Read the model definition and answer for the solid it produces. Units are mm, in the model's axes. A direction names the side the tool comes from. Coordinates: 2 decimals unless noted, no trailing zeros. Write each loop counter-clockwise with the first axis right and the second up, starting at its lowest first coordinate (ties: lowest second). Pieces come first, ordered by that corner, then holes. Notation, with made-up numbers: (-16, 69) - (30, 69) arc R28 ccw to (30, 96) - close; hole circle Ø8 at (86, -33.75). An arc over 180 degrees is marked (long way). Return JSON: item names as keys, results as strings.
```python
from build123d import *

# Parameters (mm, degrees)
SKETCH1_R           = 17.25
BOSS_EXTRUDE1_DEPTH = 4.5
SKETCH2_R           = 2
CUT_EXTRUDE1_DEPTH  = 9
SKETCH3_R           = 14.7
SKETCH3_R_2         = 6
CUT_EXTRUDE2_DEPTH  = 7
CUT_EXTRUDE3_REACH  = 4
SKETCH4_R           = 3
SKETCH5_R           = 1.35933313
CUT_EXTRUDE4_DEPTH  = 18


with BuildPart() as part:
    # Sketch1 → Boss-Extrude1 (new body, symmetric)
    with BuildSketch(Plane.XY):
        Circle(SKETCH1_R)
    extrude(amount=BOSS_EXTRUDE1_DEPTH, both=True)

    # Sketch2 → Cut-Extrude1 (cut)
    with BuildSketch(Plane.XY.offset(4.5)):
        Circle(SKETCH2_R)
    extrude(amount=-CUT_EXTRUDE1_DEPTH, mode=Mode.SUBTRACT)

    # Sketch3 → Cut-Extrude2 (cut)
    with BuildSketch(Plane.XY.offset(4.5)):
        Circle(SKETCH3_R)
        Circle(SKETCH3_R_2, mode=Mode.SUBTRACT)
    extrude(amount=-CUT_EXTRUDE2_DEPTH, mode=Mode.SUBTRACT)

    # Sketch4 → Cut-Extrude3 (cut, up to next)
    with BuildSketch(Plane.XY.offset(-2.5), mode=Mode.PRIVATE) as cut_extrude3_sk1:
        with Locations((10.5, 0)):
            Circle(SKETCH4_R)
    cut_extrude3_tool1 = extrude(cut_extrude3_sk1.sketch, amount=-CUT_EXTRUDE3_REACH, mode=Mode.PRIVATE) & part.part
    add(cut_extrude3_tool1.solids().sort_by_distance((10.5, 0, -2.5))[0], mode=Mode.SUBTRACT)
    # Sketch4 → Cut-Extrude3 (cut, up to next)
    with BuildSketch(Plane.XY.offset(-2.5), mode=Mode.PRIVATE) as cut_extrude3_sk2:
        with Locations((5.25, -9.09326674)):
            Circle(SKETCH4_R)
    cut_extrude3_tool2 = extrude(cut_extrude3_sk2.sketch, amount=-CUT_EXTRUDE3_REACH, mode=Mode.PRIVATE) & part.part
    add(cut_extrude3_tool2.solids().sort_by_distance((5.25, -9.093267, -2.5))[0], mode=Mode.SUBTRACT)
    # Sketch4 → Cut-Extrude3 (cut, up to next)
    with BuildSketch(Plane.XY.offset(-2.5), mode=Mode.PRIVATE) as cut_extrude3_sk3:
        with Locations((-5.25, -9.09326674)):
            Circle(SKETCH4_R)
    cut_extrude3_tool3 = extrude(cut_extrude3_sk3.sketch, amount=-CUT_EXTRUDE3_REACH, mode=Mode.PRIVATE) & part.part
    add(cut_extrude3_tool3.solids().sort_by_distance((-5.25, -9.093267, -2.5))[0], mode=Mode.SUBTRACT)
    # Sketch4 → Cut-Extrude3 (cut, up to next)
    with BuildSketch(Plane.XY.offset(-2.5), mode=Mode.PRIVATE) as cut_extrude3_sk4:
        with Locations((-10.5, 0)):
            Circle(SKETCH4_R)
    cut_extrude3_tool4 = extrude(cut_extrude3_sk4.sketch, amount=-CUT_EXTRUDE3_REACH, mode=Mode.PRIVATE) & part.part
    add(cut_extrude3_tool4.solids().sort_by_distance((-10.5, 0, -2.5))[0], mode=Mode.SUBTRACT)
    # Sketch4 → Cut-Extrude3 (cut, up to next)
    with BuildSketch(Plane.XY.offset(-2.5), mode=Mode.PRIVATE) as cut_extrude3_sk5:
        with Locations((-5.25, 9.09326674)):
            Circle(SKETCH4_R)
    cut_extrude3_tool5 = extrude(cut_extrude3_sk5.sketch, amount=-CUT_EXTRUDE3_REACH, mode=Mode.PRIVATE) & part.part
    add(cut_extrude3_tool5.solids().sort_by_distance((-5.25, 9.093267, -2.5))[0], mode=Mode.SUBTRACT)
    # Sketch4 → Cut-Extrude3 (cut, up to next)
    with BuildSketch(Plane.XY.offset(-2.5), mode=Mode.PRIVATE) as cut_extrude3_sk6:
        with Locations((5.25, 9.09326674)):
            Circle(SKETCH4_R)
    cut_extrude3_tool6 = extrude(cut_extrude3_sk6.sketch, amount=-CUT_EXTRUDE3_REACH, mode=Mode.PRIVATE) & part.part
    add(cut_extrude3_tool6.solids().sort_by_distance((5.25, 9.093267, -2.5))[0], mode=Mode.SUBTRACT)

    # Sketch5 → Cut-Extrude4 (cut)
    with BuildSketch(Plane(origin=(0, 0, 0), x_dir=(0, 0, -1), z_dir=(1, 0, 0))):
        Circle(SKETCH5_R)
    extrude(amount=-CUT_EXTRUDE4_DEPTH, mode=Mode.SUBTRACT)


solid = part.part
```
(1) Flat-ended cylindrical pins translate along their axes: P1, Ø5, axis at x = -12.5, z = 0, coming from the +Y side; P2, Ø4, axis at x = -7, z = 1.5, coming from the +Y side; P3, Ø4, axis at x = 6.5, z = -2.5, coming from the -Y side. Find the tip coordinate at first contact, or state that the pin passes through.
Answer:
{"P1": "y = 14.06", "P2": "y = 16.51", "P3": "y = -16.65"}
(2) A cutting plane is placed at D-D (z = 2). Determine the outline of the cut face in (x, y), and give its area (3 significant figures).
Answer:
{"outline": "circle Ø34.5 at (0, 0); circle Ø12 at (0, 0); hole circle Ø29.4 at (0, 0); hole circle Ø4 at (0, 0)", "area": "356 mm²"}
(3) Straight lines are drawn through the part: line 1 (Y direction, x = 3.5, z = 3); line 2 (Y direction, x = 5.5, z = -2); line 3 (Y direction, x = -4.75, z = 0). For each, find the intervals that lie inside material, in ascending order. Write a range as from..to.
Answer:
{"line 1": "-16.89..-14.28, -4.87..4.87, 14.28..16.89", "line 2": "-16.35..-13.63, -2.4..2.4, 13.63..16.35", "line 3": "-16.58..-13.91, -3.67..-1.36, 1.36..3.67, 13.91..16.58"}
(4) Determine the mould class of faces 1 (the face through (-3.7, 0.4, -1.3)), 2 (the face through (5.723, 1.802, 1.049)), 3 (the face through (16.453, 5.181, 0.063)) for opening direction X: +X half, -X half, draft (parallel to the pull), parting line (faces both ways), or undercut.
Answer:
{"face 1": "draft", "face 2": "undercut", "face 3": "parting line"}
(5) Which of the six approach directions +Z, -Z, +X, -X, +Y, -Y give full straight-line access (tool end or side, diameter ignored) to faces 4 (the face through (-15.925, -0.521, -1.256)), 5 (the face through (-0.2, -6.3, -2.5)), 6 (the face through (-3.64, -6.56, -3.49))?
Answer:
{"face 4": "-X", "face 5": "+Z", "face 6": "+Z, -Z"}
(6) A cutting plane is placed at A-A (x = 0). Determine the outline of the cut face in (y, z), and give its area (3 significant figures).
Answer:
{"outline": "(-17.25, -4.5) - (-2, -4.5) - (-2, 4.5) - (-6, 4.5) - (-6, -2.5) - (-14.7, -2.5) - (-14.7, 4.5) - (-17.25, 4.5) - close; (2, -4.5) - (17.25, -4.5) - (17.25, 4.5) - (14.7, 4.5) - (14.7, -2.5) - (6, -2.5) - (6, 4.5) - (2, 4.5) - close", "area": "153 mm²"}
(7) A cutting plane is placed at C-C (y = 11.5). Determine the outline of the cut face in (x, z).
Answer:
{"outline": "(-12.86, -4.5) - (-7.04, -4.5) - (-7.04, -2.5) - (-9.16, -2.5) - (-9.16, 4.5) - (-12.86, 4.5) - close; (-3.46, -4.5) - (3.46, -4.5) - (3.46, -2.5) - (-3.46, -2.5) - close; (7.04, -4.5) - (12.86, -4.5) - (12.86, 4.5) - (9.16, 4.5) - (9.16, -2.5) - (7.04, -2.5) - close"}
(8) A cutting plane is placed at B-B (z = 0). Determine the outline of the cut face in (x, y), and give its area (3 significant figures).
Answer:
{"outline": "(-17.2, -1.36) arc R17.25 ccw (long way) to (-17.2, 1.36) - (-14.64, 1.36) arc R14.7 cw (long way) to (-14.64, -1.36) - close; (-5.84, -1.36) arc R6 ccw (long way) to (-5.84, 1.36) - (-1.47, 1.36) arc R2 cw (long way) to (-1.47, -1.36) - close", "area": "338 mm²"}
